Geometry: final body of the model. Coordinates: model frame, mm. A direction names the side the tool comes from. Coordinates: 2 decimals unless noted, no trailing zeros. Loops run counter-clockwise (first coordinate to the right, second up) from the corner with the lowest first, then second, coordinate; pieces in that order, holes last. Notation, with made-up numbers: (16, 42.25) - (35, 42.25) arc R15 ccw to (35, 59.25) - close; hole circle Ø4 at (71, 23). An arc over 180 degrees is marked (long way). Return JSON: item names as keys, results as strings.
from build123d import *

# Parameters (mm, degrees)
SKETCH1_R           = 75
BOSS_EXTRUDE1_DEPTH = 5
SKETCH2_W           = 53
SKETCH2_H           = 20.734598854
BOSS_EXTRUDE2_DEPTH = 150
BOSS_EXTRUDE3_DEPTH = 53
SKETCH4_W           = 100
SKETCH4_H           = 86
BOSS_EXTRUDE4_DEPTH = 45
SHELL1_START        = -44
SHELL1_DEPTH        = 88
SHELL1_START_2      = -20.5
SHELL1_2_DEPTH      = 41
SKETCH5_W           = 88
SKETCH5_H           = 74
CUT_EXTRUDE1_DEPTH  = 10
SKETCH7_R           = 6
CUT_EXTRUDE2_DEPTH  = 10
SKETCH8_W           = 43
SKETCH8_H           = 15.969997916
CUT_EXTRUDE3_DEPTH  = 10
SKETCH10_R          = 2.65
CUT_EXTRUDE4_DEPTH  = 3
SKETCH12_W          = 15
SKETCH12_H          = 10
CUT_EXTRUDE5_DEPTH  = 10


# Read off the part's stored shape, not the designer's step: Shell1
with BuildPart() as part:
    # Sketch1 → Boss-Extrude1 (new body)
    with BuildSketch(Plane(origin=(0, 0, 0), x_dir=(1, 0, 0), z_dir=(0, 1, 0))):
        with Locations(Location((0, 0, 0), (0, 0, 270))):
            Circle(SKETCH1_R)
    extrude(amount=BOSS_EXTRUDE1_DEPTH)

    # Sketch2 → Boss-Extrude2 (add)
    with BuildSketch(Plane(origin=(0, 5, 0), x_dir=(1, 0, 0), z_dir=(0, 1, 0))):
        Rectangle(SKETCH2_W, SKETCH2_H)
    extrude(amount=BOSS_EXTRUDE2_DEPTH)

    # Sketch3 → Boss-Extrude3 (add)
    with BuildSketch(Plane.ZY.offset(26.5)):
        Polygon((-10.367299427, 155), (-10.367299427, 175.734598855), (10.367299427, 155), align=None)
    extrude(amount=-BOSS_EXTRUDE3_DEPTH)

    # Sketch4 → Boss-Extrude4 (add)
    with BuildSketch(Plane(origin=(0, 82.683649714, 82.683649714), x_dir=(1, 0, 0), z_dir=(0, 0.7071067811865513, 0.7071067811865438))):
        with Locations((0, 116.932338812)):
            Rectangle(SKETCH4_W, SKETCH4_H)
    extrude(amount=BOSS_EXTRUDE4_DEPTH)

    # Shell1 outline → Shell1 (cut)
    with BuildSketch(Plane.YZ.offset(SHELL1_START)):
        Polygon((143.446989211, 30.405591591), (195.772891018, -21.920310217), (219.107414798, 1.414213562), (166.78151299, 53.74011537), align=None)
    extrude(amount=SHELL1_DEPTH, mode=Mode.SUBTRACT)

    # Shell1 2 outline → Shell1 2 (cut)
    with BuildSketch(Plane.YZ.offset(SHELL1_START_2)):
        Polygon((6, 4.367299427), (6, -4.367299427), (178.219880229, -4.367299427), (169.485281374, 4.367299427), align=None)
    extrude(amount=SHELL1_2_DEPTH, mode=Mode.SUBTRACT)

    # Sketch5 → Cut-Extrude1 (cut)
    with BuildSketch(Plane(origin=(0, 114.503454867, 114.503454867), x_dir=(1, 0, 0), z_dir=(0, 0.7071067811865512, 0.7071067811865438))):
        with Locations((0, 116.932338812)):
            Rectangle(SKETCH5_W, SKETCH5_H)
    extrude(amount=-CUT_EXTRUDE1_DEPTH, mode=Mode.SUBTRACT)

    # Sketch7 → Cut-Extrude2 (cut)
    with BuildSketch(Plane(origin=(0, 108.846600618, -108.846600618), x_dir=(1, 0, 0), z_dir=(0, -0.7071067811865438, 0.7071067811865512))):
        with Locations(Location((36.5, 141.33938714, 0), (0, 0, 270))):
            Circle(SKETCH7_R)
    extrude(amount=-CUT_EXTRUDE2_DEPTH, mode=Mode.SUBTRACT)

    # Sketch8 → Cut-Extrude3 (cut)
    with BuildSketch(Plane(origin=(0, 0, -10.367299427), x_dir=(-1, 0, 0), z_dir=(0, 0, -1))):
        with Locations((0, 20.660666548)):
            Rectangle(SKETCH8_W, SKETCH8_H)
    extrude(amount=-CUT_EXTRUDE3_DEPTH, mode=Mode.SUBTRACT)

    # Sketch10 → Cut-Extrude4 (cut)
    with BuildSketch(Plane(origin=(0, 114.503454867, 114.503454867), x_dir=(1, 0, 0), z_dir=(0, 0.7071067811865512, 0.7071067811865438))):
        with Locations(Location((-47, 76.932338812, 0), (0, 0, 270))):
            Circle(SKETCH10_R)
        with Locations(Location((-47, 156.932338812, 0), (0, 0, 270))):
            Circle(SKETCH10_R)
        with Locations(Location((47, 76.932338812, 0), (0, 0, 270))):
            Circle(SKETCH10_R)
        with Locations(Location((47, 156.932338812, 0), (0, 0, 270))):
            Circle(SKETCH10_R)
    extrude(amount=-CUT_EXTRUDE4_DEPTH, mode=Mode.SUBTRACT)

    # Sketch12 → Cut-Extrude5 (cut)
    with BuildSketch(Plane(origin=(0, 108.846600618, -108.846600618), x_dir=(1, 0, 0), z_dir=(0, -0.7071067811865438, 0.7071067811865512))):
        with Locations((-10.5, 151.932338812)):
            Rectangle(SKETCH12_W, SKETCH12_H)
    extrude(amount=-CUT_EXTRUDE5_DEPTH, mode=Mode.SUBTRACT)


solid = part.part
Item 1: Ray query, probe 1 along Z at (x, y) = (-15.5, 80.5); probe 2 along Y at (x, z) = (-27.5, -29); probe 3 along Y at (x, z) = (-19.5, -25). Return the intervals inside material, ascending. Write a range as from..to.
Worked out:
{"probe 1": "-10.37..-4.37, 4.37..10.37", "probe 2": "0..5, 194.37..197.18", "probe 3": "0..5, 190.37..201.18"}
Item 2: Reachability of faces 4 (the face through (-0.62, 157.43, 44.39)), 5 (the face through (-21.5, 21, -5)), 6 (the face through (26.5, 92, 0)), 7 (the face through (-44, 183, 19)) from +Z, -Z, +X, -X, +Y, -Y: full face, straight path, thin tool, end or side. Return the list, or none.
Worked out:
{"face 4": "+Y", "face 5": "-Z", "face 6": "-Z, +X", "face 7": "none"}
Item 3: Section query A-A, the plane x = 0. Return loops of the section in (y, z), and give its area (3 significant figures).
Worked out:
{"outline": "(0, -75) - (5, -75) - (5, -10.37) - (12.68, -10.37) - (12.68, -4.37) - (6, -4.37) - (6, 4.37) - (169.49, 4.37) - (143.45, 30.41) - (171.02, 57.98) - (166.78, 62.23) - (134.96, 30.41) - (155, 10.37) - (5, 10.37) - (5, 75) - (0, 75) - close; (28.65, -10.37) - (175.73, -10.37) - (195.77, -30.41) - (227.59, 1.41) - (223.35, 5.66) - (195.77, -21.92) - (178.22, -4.37) - (28.65, -4.37) - close", "area": "3,500 mm^2"}
Item 4: First-contact query: pin 1 Ø4.5 at (y, z) = (63, 0) entering from -X; pin 2 Ø6 at (y, z) = (66, 0) entering from +X; pin 3 Ø1 at (x, y) = (13.5, 203) entering from +Z; pin 4 Ø5 at (x, z) = (37.5, 55.5) entering from -Y. Flat tips, straight axial feed; report the tip coordinate or a pass-through.
Worked out:
{"pin 1": "x = -26.5", "pin 2": "x = 26.5", "pin 3": "z = -14.19", "pin 4": "y = 0"}
Item 5: Section query B-B, the plane y = 101.5. Return loops of the section in (x, z), and give its area (3 significant figures).
Worked out:
{"outline": "(-26.5, -10.37) - (26.5, -10.37) - (26.5, 10.37) - (-26.5, 10.37) - close; hole (-20.5, -4.37) - (20.5, -4.37) - (20.5, 4.37) - (-20.5, 4.37) - close", "area": "741 mm^2"}
Item 6: Mould query, pull axis X, two halves, no side actions, for faces 1 (the face through (-50, 181, 16)), 2 (the face through (0, 12.676, -8)), 3 (the face through (1, 5, 16)). Classes: +X half, -X half, draft (parallel to the pull), parting line (faces both ways), or undercut.
Worked out:
{"face 1": "-X half", "face 2": "undercut", "face 3": "draft"}
Item 7: Section query C-C, the plane z = 45. Return loops of the section in (x, y).
Worked out:
{"outline": "(-60, 0) - (60, 0) - (60, 5) - (-60, 5) - close; (-50, 149.56) - (50, 149.56) - (50, 184.01) - (44, 184.01) - (44, 158.04) - (-44, 158.04) - (-44, 184.01) - (-50, 184.01) - close"}
Item 8: Section query D-D, the plane x = -30. Return loops of the section in (y, z).
Worked out:
{"outline": "(0, -68.74) - (5, -68.74) - (5, 68.74) - (0, 68.74) - close; (134.96, 30.41) - (195.77, -30.41) - (227.59, 1.41) - (223.35, 5.66) - (195.77, -21.92) - (143.45, 30.41) - (171.02, 57.98) - (166.78, 62.23) - close"}
